CAD build for the part. Positions are in the model's coordinates, mm. A direction names the side the tool comes from. Coordinates: 2 decimals unless noted, no trailing zeros. Loops run counter-clockwise (first coordinate to the right, second up) from the corner with the lowest first, then second, coordinate; pieces in that order, holes last. Notation, with made-up numbers: (11.25, 18.5) - (50.25, 18.5) arc R29 ccw to (50.25, 47.5) - close; hole circle Ø11 at (16.25, 70.5). An arc over 180 degrees is marked (long way). Put each result on its own line as item: value.
```python
from build123d import *

# Parameters (mm, degrees)
F0_W      = 60
F0_H      = 33.1892187767
F1_DEPTH  = 40
F3_DEPTH  = 41.91
F5_DEPTH  = 30
F6_DEPTH  = 20
F8_DEPTH  = 25.4
F10_DEPTH = 25.4


with BuildPart() as f1:
    # F0 (on Front) → F1 (new body)
    with BuildSketch(Plane.XZ):
        with Locations((-30, -16.5946093883)):
            Rectangle(F0_W, F0_H)
    extrude(amount=F1_DEPTH)

    # F2 (on Front) → F3 (cut)
    with BuildSketch(Plane.XZ):
        Polygon((0, -20), (0, 0), (-19.5117478243, 0), align=None)
    extrude(amount=F3_DEPTH, mode=Mode.SUBTRACT)

    # F4 (on face) → F5 (cut)
    with BuildSketch(Plane(origin=(0, 0, 0), x_dir=(-1, 0, 0), z_dir=(0, 1, 0))):
        Polygon((0, -20), (0, -26.5946093883), (50, -26.5946093883), (50, -33.1892187767), (60, -33.1892187767), (60, -6.581982132), (30, -6.581982132), (30, 0), (19.5117478243, 0), align=None)
    extrude(amount=-F5_DEPTH, mode=Mode.SUBTRACT)

    # F6 (cut): a face of the model
    f6_faces = [f1.faces().sort_by_distance(p)[0] for p in [
        (-45, 0, -3.290991066),
    ]]
    extrude(f6_faces, amount=-F6_DEPTH, mode=Mode.SUBTRACT)

    # F7 (on face) → F8 (cut)
    with BuildSketch(Plane.XY.offset(-26.5946093883)):
        Polygon((-50, 0), (-50, -30), (-30.9202261269, 0), align=None)
    extrude(amount=-F8_DEPTH, mode=Mode.SUBTRACT)

    # F9 (on face) → F10 (cut)
    with BuildSketch(Plane(origin=(0, 0, -33.1892187767), x_dir=(1, 0, 0), z_dir=(0, 0, -1))):
        Polygon((-25.575999478, 16.2872133739), (-16.1481829174, 16.2872133739), (-16.1481829174, 25.2565963231), (-26.1481829174, 25.2565963231), align=None)
    extrude(amount=-F10_DEPTH, mode=Mode.SUBTRACT)


solid = f1.part
```
Q1. Slice it at A-A, the plane z = -30.5. Give the cut face in (x, y), then the cut area to 3 significant figures.
Determined:
outline: (-60, -40) - (0, -40) - (0, 0) - (-30.92, 0) - (-50, -30) - (-60, -30) - close; hole (-26.15, -25.26) - (-16.15, -25.26) - (-16.15, -16.29) - (-25.58, -16.29) - close
area: 1,730 mm2
Q2. Slice it at D-D, the plane x = -39.5. Give the cut face in (y, z), then the cut area to 3 significant figures.
Determined:
outline: (-40, -33.19) - (-13.49, -33.19) - (-13.49, -26.59) - (-30, -26.59) - (-30, -6.58) - (-20, -6.58) - (-20, 0) - (-40, 0) - close
area: 507 mm2
Q3. Tool access for faces 5 (the flat face through (-16.148, -21, -30)), 6 (the flat face through (-30, -40, -16)), 7 (the flat face through (-30, -25, -3)), 8 (the flat face through (-19, -15, -26.595)), 9 (the flat face through (-45, -20, -3)): list every direction of +Z, -Z, +X, -X, +Y, -Y with a clear straight run to the whole face (end or side of a thin tool).
Determined:
face 5: +Z, -Z
face 6: +Z, -Z, +X, -X, -Y
face 7: +Z, +X, +Y
face 8: +X, -X, +Y
face 9: +Z, +X, -X, +Y
Q4. Slice it at B-B, the plane y = -36. Give the cut face in (x, z).
Determined:
outline: (-60, -33.19) - (0, -33.19) - (0, -20) - (-19.51, 0) - (-60, 0) - close
Q5. Mould opens along Y. For faces 1 (the flat face through (-60, -34, -13)), 2 (the flat face through (-25.866, -20.835, -29.938)), 3 (the flat face through (-40.594, -15.21, -29.846)), 4 (the flat face through (-21, -16.287, -30)) say: +Y half, -Y half, draft (parallel to the pull), parting line (faces both ways), or undercut.
Determined:
face 1: draft
face 2: undercut
face 3: +Y half
face 4: undercut
Q6. Wall check: L1, parallel to Z at x = -49, y = -27; L2, parallel to Y at x = -31, z = -5.5; L3, parallel to X at y = -24, z = -6.5. Give the ranges that are in metal, low to high. Write a range as from..to.
Determined:
L1: -6.58..0
L2: -40..-20
L3: -60..-30
Q7. Pin check, flat tips, straight feed: pin 1 Ø8 at (x, y) = (-48.5, -25.5) entering from -Z; pin 2 Ø7 at (x, z) = (-48, -2) entering from +Y; pin 3 Ø3 at (x, z) = (-35.5, -23) entering from +Y; pin 4 Ø3 at (x, y) = (-25.5, -8) entering from +Z. Stop position of each tip, or through.
Determined:
pin 1: z = -33.19
pin 2: y = -20
pin 3: y = -30
pin 4: z = -26.59
Q8. Slice it at C-C, the plane y = -18. Give the cut face in (x, z).
Determined:
outline: (-42.37, -33.19) - (-25.69, -33.19) - (-25.69, -26.59) - (-42.37, -26.59) - close; (-16.15, -33.19) - (0, -33.19) - (0, -26.59) - (-16.15, -26.59) - close
